Could you check a few things on this model? Use its own coordinates, in mm. A direction names the side the tool comes from. Give positions to 0.01 mm unless a question says otherwise; leave off trailing zeros. Loops run counter-clockwise (first coordinate to the right, second up) from the corner with the lowest first, then second, coordinate; pieces in that order, holes last. Notation, with made-up numbers: (24, -13.5) - (28, -13.5) arc R16 ccw to (28, -4.5) - close; hole circle Ø1 at (-5, 72.25). An arc over 180 degrees is marked (long way). Write each question's results on one line, items separated by ' | '. Start each with the question number.
1) I'm going to push flat-ended pins straight in: pin 1 (8 mm diameter, centred on y = 9.5, z = 32.5, fed in from -X); pin 2 (3 mm diameter, centred on x = 13.42, y = -7.75, fed in from +Z); pin 3 (5 mm diameter, centred on y = 6, z = 42, fed in from +X); pin 4 (2 mm diameter, centred on y = 8.5, z = -6.5, fed in from +X) (3 decimals). Where does each tip first touch, or does it pass through?
2) I want a section at C-C, the plane x = -7. Write out the boundary of the cut face in (y, z).
3) On a 3-axis mill with a long thin cutter (end or side, diameter ignored), from which of +Z, -Z, +X, -X, +Y, -Y can I reach the whole of each face in a straight line? I mean faces 1 (the face through (-7, 0, -22.86)), 2 (the face through (10, 0, 55)), 3 (the face through (-11, 0, 55)), 4 (the face through (-0.16, -14.26, 1.52)), 5 (the face through (-4.6, 0, -17)). Say none if no direction works.
4) I want a section at B-B, the plane z = 9. Write out the boundary of the cut face in (x, y), and give its area (3 significant figures).
5) If I drill on probe 1 along Y at (x, z) = (0, 2); probe 2 along X at (y, z) = (-7.75, 1.8); probe 3 along Z at (x, y) = (1, -13.5), over which ranges is the centre line in solid material (lowest first)? Write a range as [from, to].
6) If we mould it in two halves opening along Y, with no side actions, what happens to faces 6 (the face through (-12.27, -8.23, 1.52)), 7 (the face through (-10, 0, 55)), 8 (the face through (-10, 0, -14))? For each: +Y half, -Y half, draft (parallel to the pull), parting line (faces both ways), or undercut.
from build123d import *

# Parameters (mm, degrees)
SKETCH1_R                   = 17.272
BOSS_EXTRUDE1_DEPTH         = 52.22
SKETCH1_3_R                 = 6
BOSS_EXTRUDE2_DEPTH         = 6.5
BOSS_EXTRUDE3_DEPTH         = 22.86
SKETCH1_5_R                 = 3
BOSS_EXTRUDE4_DEPTH         = 10.668
SKETCH2_W                   = 1
SKETCH2_H                   = 5
BOSS_EXTRUDE5_DEPTH         = 6
SKETCH4_R                   = 18.4
BOSS_EXTRUDE6_DEPTH         = 22
TAP_DRILL_FOR_M3_TAP1_D     = 2.5
TAP_DRILL_FOR_M3_TAP1_DEPTH = 3
TAP_DRILL_FOR_M3_TAP1_TIP   = 0.751075774
CHAMFER1_SIZE               = 0.2
CHAMFER2_SIZE               = 0.5


with BuildPart() as part:
    # Sketch1 → Boss-Extrude1 (new body)
    with BuildSketch(Plane.XY):
        Circle(SKETCH1_R)
    extrude(amount=BOSS_EXTRUDE1_DEPTH)

    # Sketch1_3 → Boss-Extrude2 (add)
    with BuildSketch(Plane.XY):
        with Locations((-7, 0)):
            Circle(SKETCH1_3_R)
    extrude(amount=-BOSS_EXTRUDE2_DEPTH)

    # Sketch1_4 → Boss-Extrude3 (add)
    with BuildSketch(Plane.XY):
        with BuildLine():
            Line((-4.6, -1.8), (-4.6, 1.8))
            ThreePointArc((-4.6, 1.8), (-10, 0), (-4.6, -1.8))
        make_face()
    extrude(amount=-BOSS_EXTRUDE3_DEPTH)

    # Sketch1_5 → Boss-Extrude4 (add)
    with BuildSketch(Plane.XY):
        with Locations((-7, 0)):
            Circle(SKETCH1_5_R)
    extrude(amount=-BOSS_EXTRUDE4_DEPTH)

    # Sketch2 → Boss-Extrude5 (add)
    with BuildSketch(Plane.XY.offset(52.22)):
        with Locations((-10.5, 0)):
            Rectangle(SKETCH2_W, SKETCH2_H)
        with Locations((10.5, 0)):
            Rectangle(SKETCH2_W, SKETCH2_H)
    extrude(amount=BOSS_EXTRUDE5_DEPTH)

    # Sketch4 → Boss-Extrude6 (add)
    with BuildSketch(Plane(origin=(0, 0, 0), x_dir=(-1, 0, 0), z_dir=(0, 0, -1))):
        Circle(SKETCH4_R)
    extrude(amount=-BOSS_EXTRUDE6_DEPTH)

    # Tap Drill for M3 Tap1
    with Locations(Plane(origin=(0, 0, 0), x_dir=(-1, 0, 0), z_dir=(0, 0, -1))):
        with Locations((-13.423393759, -7.75), (0, -15.5), (0, 15.5), (13.423393759, 7.75), (13.423393759, -7.75), (-13.423393759, 7.75)):
            Hole(TAP_DRILL_FOR_M3_TAP1_D / 2, depth=TAP_DRILL_FOR_M3_TAP1_DEPTH)
            with Locations((0, 0, -(TAP_DRILL_FOR_M3_TAP1_DEPTH + TAP_DRILL_FOR_M3_TAP1_TIP / 2))):  # 118° drill point
                Cone(0, TAP_DRILL_FOR_M3_TAP1_D / 2, TAP_DRILL_FOR_M3_TAP1_TIP, mode=Mode.SUBTRACT)

    # Chamfer1
    chamfer1_edges = [part.edges().sort_by_distance(p)[0] for p in [
        (-10, 0, -22.86),
    ]]
    chamfer(chamfer1_edges, length=CHAMFER1_SIZE)

    # Chamfer2
    chamfer2_edges = [part.edges().sort_by_distance(p)[0] for p in [
        (-13, 0, -6.5),
    ]]
    chamfer(chamfer2_edges, length=CHAMFER2_SIZE)


solid = part.part
Answers:
1) pin 1: stops at x = -16.37 | pin 2: stops at z = 52.22 | pin 3: stops at x = 16.91 | pin 4: passes through
2) outline: (-17.02, 0) - (-6, 0) - (-6, -6) - (-5.5, -6.5) - (-3, -6.5) - (-3, -22.66) - (-2.8, -22.86) - (2.8, -22.86) - (3, -22.66) - (3, -6.5) - (5.5, -6.5) - (6, -6) - (6, 0) - (17.02, 0) - (17.02, 22) - (15.79, 22) - (15.79, 52.22) - (-15.79, 52.22) - (-15.79, 22) - (-17.02, 22) - close
3) face 1: -Z, +X, -X, +Y, -Y | face 2: +Z, +Y, -Y | face 3: +Z, -X, +Y, -Y | face 4: -Z | face 5: -Z, +X, +Y, -Y
4) outline: circle Ø36.8 at (0, 0) | area: 1,060 mm2
5) probe 1: y = [-18.4, -16.75], [-14.25, 14.25], [16.75, 18.4] | probe 2: x = [-16.69, -14.67], [-12.17, 12.17], [14.67, 16.69] | probe 3: z = [0, 52.22]
6) face 6: undercut | face 7: draft | face 8: parting line
